The listing builds one solid part. Answer for the finished solid, in the listing's coordinates (mm). A direction names the side the tool comes from. Round coordinates to 2 decimals unless told otherwise and drop trailing zeros. Loops run counter-clockwise (first coordinate to the right, second up) from the corner with the lowest first, then second, coordinate; pieces in that order, holes last. Notation, with made-up numbers: (47.25, 42.5) - (97.25, 42.5) arc R21 ccw to (97.25, 76.5) - close; hole circle Ø6 at (-38.5, -17.5). An arc over 180 degrees is marked (long way). One line per item, written item: value.
```python
from build123d import *

# Parameters (mm, degrees)
F0_R     = 12.7
F1_DEPTH = 1200
F2_R     = 12.7
F3_DEPTH = 40
F4_DEPTH = 200


with BuildPart() as f1:
    # F0 (on Right) → F1 (new body)
    with BuildSketch(Plane.YZ):
        Circle(F0_R)
    extrude(amount=-F1_DEPTH)

    # F2 (on Top) → F3 (join)
    with BuildSketch(Plane.XY):
        with Locations((-850, 0)):
            Circle(F2_R)
    extrude(amount=-F3_DEPTH)

    # F4 (add): a face of the model
    f4_faces = [f1.faces().sort_by_distance(p)[0] for p in [
        (0, 0, 0),
    ]]
    extrude(f4_faces, amount=F4_DEPTH)


solid = f1.part
```
1) A cutting plane is placed at B-B on x = -850. Give the vertices of the cut face in (y, z), and give its area (3 significant figures).
Final values:
outline: (-12.7, -40) - (12.7, -40) - (12.7, 0) arc R12.7 ccw to (-12.7, 0) - close
area: 1,270 mm2
2) Consider L1, parallel to X at y = -0.5, z = -17.5; L2, parallel to X at y = 2, z = -25.5; L3, parallel to Z at x = -355, y = 0.5. Determine where each line is inside the solid, lowest interval first.
Final values:
L1: -862.69 to -837.31
L2: -862.54 to -837.46
L3: -12.69 to 12.69
3) A cutting plane is placed at D-D on x = -665.5. Give the vertices of the cut face in (y, z).
Final values:
outline: circle Ø25.4 at (0, 0)
4) A cutting plane is placed at A-A on y = 0. Give the vertices of the cut face in (x, z).
Final values:
outline: (-1200, -12.7) - (-862.7, -12.7) - (-862.7, -40) - (-837.3, -40) - (-837.3, -12.7) - (200, -12.7) - (200, 12.7) - (-1200, 12.7) - close
5) A cutting plane is placed at C-C on z = -21.5. Give the vertices of the cut face in (x, y).
Final values:
outline: circle Ø25.4 at (-850, 0)
6) For faces 1 (the cylindrical face through (-862.688, 0.558, -24.164)), 2 (the flat face through (200, 0, 0)), determine the directions among +Z, -Z, +X, -X, +Y, -Y from which every point of the face is accessible in a straight line to the end or side of a thin tool.
Final values:
face 1: -Z
face 2: +Z, -Z, +X, +Y, -Y
7) Each of these flat-tipped pins is pushed along its axis until it touches: pin 1 Ø12 at (x, z) = (-243.5, -21.5) entering from -Y; pin 2 Ø8 at (y, z) = (-6, -34.5) entering from +X; pin 3 Ø10 at (x, y) = (-453.5, 7) entering from -Z; pin 4 Ø1 at (x, y) = (-1059, -1.5) entering from -Z. Where does it stop, or does it pass through?
Final values:
pin 1: through
pin 2: x = -837.46
pin 3: z = -12.54
pin 4: z = -12.66
